```python
from build123d import *

# Parameters (mm, degrees)
F0_W     = 25.4
F0_H     = 127
F1_DEPTH = 1.5875
F2_R     = 9.525
F3_DEPTH = 25.4
F4_R     = 9.525
F5_DEPTH = 25.4
F6_R     = 9.525
F7_DEPTH = 25.4
F8_R     = 9.525
F9_DEPTH = 25.4


with BuildPart() as f1:
    # F0 (on Front) → F1 (new body, symmetric)
    with BuildSketch(Plane.XZ):
        Rectangle(F0_W, F0_H)
    extrude(amount=F1_DEPTH, both=True)

    # F2 (on face) → F3 (cut)
    with BuildSketch(Plane.XZ.offset(1.5875)):
        with Locations((0, 50.328158)):
            Circle(F2_R)
    extrude(amount=-F3_DEPTH, mode=Mode.SUBTRACT)

    # F4 (on face) → F5 (cut)
    with BuildSketch(Plane.XZ.offset(1.5875)):
        with Locations((0, -50.553336)):
            Circle(F4_R)
    extrude(amount=-F5_DEPTH, mode=Mode.SUBTRACT)

    # F6 (on face) → F7 (cut)
    with BuildSketch(Plane.XZ.offset(1.5875)):
        Circle(F6_R)
    extrude(amount=-F7_DEPTH, mode=Mode.SUBTRACT)

    # F8 (on face) → F9 (cut)
    with BuildSketch(Plane.XZ.offset(1.5875)):
        with Locations((0, -25.097863)):
            Circle(F8_R)
    extrude(amount=-F9_DEPTH, mode=Mode.SUBTRACT)


solid = f1.part
```
Design review of the part built by this model. Coordinates are the model's own, in mm. Give positions to 0.01 mm unless a question says otherwise; leave off trailing zeros. Loops run counter-clockwise (first coordinate to the right, second up) from the corner with the lowest first, then second, coordinate; pieces in that order, holes last. Notation, with made-up numbers: M 7,82.5 L 18,82.5 A7 cw 18,93.5 Z; hole C 68,13.25 d9. An arc over 180 degrees is marked long. Return JSON: item names as keys, results as strings. Group by question number.
Item 1: We need section C-C (y = -0.35). Give the boundary of the cut face in (x, z) (3 decimals).
Item 2: We need section D-D (x = 0). Give the boundary of the cut face in (y, z) (1 decimal).
Item 3: We need section B-B (x = 6.5). Give the boundary of the cut face in (y, z).
Item 4: We need section A-A (z = 0). Give the boundary of the cut face in (x, y) (1 decimal).
Item 5: Insertion check: pin 1 Ø11.5 at (x, z) = (0, 50.33) entering from +Y. The pin has a flat end and moves straight along its axis. Give the tip position at first contact, or say it passes through.
Item 6: For probe 1 along Z at (x, y) = (0, 0.9) (3 decimals); probe 2 along Z at (x, y) = (2.75, -1.3); probe 3 along X at (y, z) = (1.2, -4), list the stretches that pass through material, from the lowest coordinate up.
Output:
{
 "1": {"outline": "M -12.7,-63.5 L 12.7,-63.5 L 12.7,63.5 L -12.7,63.5 Z; hole C 0,-50.553 d19.05; hole C 0,-25.098 d19.05; hole C 0,0 d19.05; hole C 0,50.328 d19.05"},
 "2": {"outline": "M -1.6,-63.5 L 1.6,-63.5 L 1.6,-60.1 L -1.6,-60.1 Z; M -1.6,-41 L 1.6,-41 L 1.6,-34.6 L -1.6,-34.6 Z; M -1.6,-15.6 L 1.6,-15.6 L 1.6,-9.5 L -1.6,-9.5 Z; M -1.6,9.5 L 1.6,9.5 L 1.6,40.8 L -1.6,40.8 Z; M -1.6,59.9 L 1.6,59.9 L 1.6,63.5 L -1.6,63.5 Z"},
 "3": {"outline": "M -1.59,-63.5 L 1.59,-63.5 L 1.59,-57.52 L -1.59,-57.52 Z; M -1.59,-43.59 L 1.59,-43.59 L 1.59,-32.06 L -1.59,-32.06 Z; M -1.59,-18.14 L 1.59,-18.14 L 1.59,-6.96 L -1.59,-6.96 Z; M -1.59,6.96 L 1.59,6.96 L 1.59,43.37 L -1.59,43.37 Z; M -1.59,57.29 L 1.59,57.29 L 1.59,63.5 L -1.59,63.5 Z"},
 "4": {"outline": "M -12.7,-1.6 L -9.5,-1.6 L -9.5,1.6 L -12.7,1.6 Z; M 9.5,-1.6 L 12.7,-1.6 L 12.7,1.6 L 9.5,1.6 Z"},
 "5": {"pin 1": "passes through"},
 "6": {"probe 1": "z = -63.5 to -60.078, -41.028 to -34.623, -15.573 to -9.525, 9.525 to 40.803, 59.853 to 63.5", "probe 2": "z = -63.5 to -59.67, -41.43 to -34.22, -15.98 to -9.12, 9.12 to 41.21, 59.45 to 63.5", "probe 3": "x = -12.7 to -8.64, 8.64 to 12.7"}
}
